Autodesk Inventor part; units mm, degrees
ref_plane "YZ Plane" through (0, 0, 0) normal (1, 0, 0) x (0, 1, 0)
ref_plane "XZ Plane" through (0, 0, 0) normal (0, 1, 0) x (-1, 0, 0)
ref_plane "XY Plane" through (0, 0, 0) normal (0, 0, 1) x (1, 0, 0)
sketch "Sketch1" plane through (0, 0, 0) normal (0, 1, 0) x (-1, 0, 0)
  line L0 (0, 0) -> (9.1604, 0) construction
  line L1 (9.1604, 0) -> (15.24, 0)
  line L2 (15.24, 0) -> (15.24, 6.35)
  line L3 (15.24, 6.35) -> (13.97, 6.35)
  line L4 (13.97, 6.35) -> (13.97, 10.922)
  line L5 (13.97, 10.922) -> (8.8191, 10.922)
  line L6 (8.8191, 10.922) -> (9.1604, 0)
  line L7 (0, 0) -> (0, 10.922)
  line L8 (0, 10.922) -> (8.8191, 10.922) construction
  line L9 (0, 0) -> (0, 28.448) construction
  line L10 (0, 28.448) -> (-17.526, 28.448) construction
  arc A0 (0, 10.922) -> (-17.526, 28.448) centre (-17.526, 10.922) ccw
  line L11 (-17.526, 28.448) -> (-28.7343, 28.448)
  line L12 (-28.448, 37.6084) -> (-28.448, 43.688)
  line L13 (-28.448, 43.688) -> (-22.098, 43.688)
  line L14 (-17.526, 42.418) -> (-17.526, 37.2671)
  line L15 (-17.526, 37.2671) -> (-17.526, 28.448) construction
  line L16 (-22.098, 43.688) -> (-22.098, 42.418)
  line L17 (-22.098, 42.418) -> (-17.526, 42.418)
  line L18 (-17.526, 37.2671) -> (-28.448, 37.6084)
  line L19 (-28.448, 37.6084) -> (-28.7343, 28.448) construction
  dimension "d0" = 18.3208
  dimension "d1" = 27.94
  dimension "d2" = 30.48
  dimension "d3" = 6.35
  dimension "d4" = 10.922
  dimension "d5" = 1.79
  dimension "d8" = 90
  dimension "d9" = 28.448
  dimension "d10" = 17.526
  dimension "d12" = 1.79
  dimension "d13" = 10.922
  dimension "d14" = 6.35
  dimension "d15" = 18.3208
  dimension "d17" = 27.94
  dimension "d18" = 30.48
revolve "Revolution1" add sketch "Sketch1" angle 360 about axis through (0, 0, 0) along (0, 0, 1) contours L6 L5 L4 L3 L2 L1
sketch "Sketch3" plane through (0, 0, 10.922) normal (0, 0, 1) x (1, 0, 0)
  circle A0 centre (0, 0) radius 11.43
  circle A1 centre (0, 0) radius 13.97
  circle A2 centre (0, 0) radius 13.97
  dimension "d6" = 22.86
  dimension "d7" = 27.94
sweep "Sweep1" add profiles "Sketch3" path "Sketch1" path curves A0
revolve "Revolution2" add sketch "Sketch1" angle 360 about axis through (17.526, 0, 28.448) along (1, 0, 0) contours L12 L13 L16 L17 L14 L18
thread "Thread1"
thread "Thread2"
equation "\"d0\" = MD"
equation "\"d1\" = F1 + 2 * G"
equation "\"d2\" = H"
equation "\"d3\" = E1"
equation "\"d4\" = B"
equation "\"d9\" = A"
equation "\"d10\" = A - B"
equation "\"d13\" = B"
equation "\"d14\" = E1"
equation "\"d15\" = MD"
equation "\"d17\" = F1 + 2 * G"
equation "\"d18\" = H"
equation "\"d6\" = F1"
equation "\"d7\" = F1 + 2 * G"
equation "\"d58\" = B"
equation "\"MD\" = 18.32077"
equation "\"A\" = 28.448"
equation "\"B\" = 10.922"
equation "\"G\" = 2.54"
equation "\"F1\" = 22.86"
equation "\"P\" = 1.8143"
equation "\"H\" = 30.48"
equation "\"E1\" = 6.35"
equation "\"Size_Designation\" = 0.5"
properties part number "ASME B16.3 90 Deg Elbow - Class 150 1/2" material "Iron, Malleable"
Check sheet for the modelled part. Datum: model origin and axes. Units: mm. A direction names the side the tool comes from. Give positions to 0.01 mm unless a question says otherwise; leave off trailing zeros. Loops run counter-clockwise (first coordinate to the right, second up) from the corner with the lowest first, then second, coordinate; pieces in that order, holes last. Notation, with made-up numbers: M 15,-35.75 L 52,-35.75 A19 ccw 52,-22.75 Z; hole C 64.25,63 d6. An arc over 180 degrees is marked long. Answer in a Markdown table with one row per item.
1) Cross-section at A-A (y = 0). Enter the section's corners in (x, z), plus the area to 3 significant figures.
Solutions:
| item | result |
|---|---|
| outline | M -15.24,0 L -9.16,0 L -8.82,10.92 L -11.43,10.92 A28.96 cw 17.53,39.88 L 17.53,37.27 L 28.45,37.61 L 28.45,43.69 L 22.1,43.69 L 22.1,42.42 L 17.53,42.42 A31.5 ccw -13.97,10.92 L -13.97,6.35 L -15.24,6.35 Z; M 8.82,10.92 L 9.16,0 L 15.24,0 L 15.24,6.35 L 13.97,6.35 L 13.97,10.92 A3.56 cw 17.53,14.48 L 22.1,14.48 L 22.1,13.21 L 28.45,13.21 L 28.45,19.29 L 17.53,19.63 L 17.53,17.02 A6.1 ccw 11.43,10.92 Z |
| area | 390 mm^2 |
2) Depth check by flat-ended pin: pin 1 (1 mm diameter, centred on x = -4.5, z = 9.5, fed in from -Y); pin 2 (10 mm diameter, centred on x = 2, z = 13.5, fed in from +Y); pin 3 (4 mm diameter, centred on x = 17, z = 22, fed in from +Y). Enter the tip coordinate at first touch or a pass-through.
Solutions:
| item | result |
|---|---|
| pin 1 | stops at y = -13.39 |
| pin 2 | stops at y = 13.97 |
| pin 3 | stops at y = 13.25 |
3) Cross-section at B-B (z = 3). Enter the section's corners in (x, y), plus the area to 3 significant figures.
Solutions:
| item | result |
|---|---|
| outline | C 0,0 d30.48; hole C 0,0 d18.13 |
| area | 471 mm^2 |
4) Thickness scan on line 1 (Y direction, x = 8.5, z = 25.5); line 2 (Z direction, x = -9.5, y = -10.5); line 3 (Z direction, x = 6.5, y = -8). Record the ranges inside material, lowest first.
Solutions:
| item | result |
|---|---|
| line 1 | y = -13.96 to -11.42, 11.42 to 13.96 |
| line 2 | z = 0 to 6.35 |
| line 3 | z = 0 to 10.92, 34.13 to 37.72 |
5) Mould release check, pull along Z, two halves, no side actions. Record for faces 1 (the face through (28.448, 7, 35)), 2 (the face through (-13.5, 4.4, 6.35)), 3 (the face through (25.23, -9.27, 16.35)): released by +Z, released by -Z, zero draft, split by the parting line, or undercut.
Solutions:
| item | result |
|---|---|
| face 1 | zero draft |
| face 2 | undercut |
| face 3 | split by the parting line |
6) Tool access check on faces 4 (the face through (17.526, 8.4, 31.8)), 5 (the face through (23.063, -0.395, 19.465)), 6 (the face through (1.95, -8.78, 5.38)), 7 (the face through (-7, 7, 0)). Record the directions out of +Z, -Z, +X, -X, +Y, -Y that give a thin tool (end or side, any length) a straight path to the whole face; none if there is none.
Solutions:
| item | result |
|---|---|
| face 4 | none |
| face 5 | +X |
| face 6 | -Z |
| face 7 | -Z, +X, -X, +Y, -Y |
